Can you work these out from the model? Positions are in its coordinate system, mm. A direction names the side the tool comes from. Round coordinates to 2 decimals unless told otherwise and drop trailing zeros. Order: outer loops, then holes, each group sorted by start corner. A loop starts at its lowest first (then second) coordinate and runs counter-clockwise, first axis right, second up. Notation, with made-up numbers: M 53,84.5 L 80,84.5 A21 ccw 80,123.5 Z; hole C 58,66 d4. An arc over 180 degrees is marked long. Answer as a JSON object with one key per item and string values. Group by question number.
from build123d import *

# Parameters (mm, degrees)
SKETCH1_R          = 2.725
EXTRUDE1_DEPTH     = 2
CUT_EXTRUDE1_DEPTH = 1
SKETCH3_R          = 1.5
EXTRUDE2_DEPTH     = 20


with BuildPart() as part:
    # Sketch1 → Extrude1 (new body)
    with BuildSketch(Plane.XY):
        Circle(SKETCH1_R)
    extrude(amount=EXTRUDE1_DEPTH)

    # Sketch2 → Cut-Extrude1 (cut)
    with BuildSketch(Plane(origin=(0, 0, 0), x_dir=(-1, 0, 0), z_dir=(0, 0, -1))):
        Polygon((3.449801909, 0), (3.449801909, 0.55), (-3.901269584, 0.55), (-3.901269584, -0.55), (3.449801909, -0.55), align=None)
    extrude(amount=-CUT_EXTRUDE1_DEPTH, mode=Mode.SUBTRACT)

    # Sketch3 → Extrude2 (add)
    with BuildSketch(Plane.XY.offset(2)):
        Circle(SKETCH3_R)
    extrude(amount=EXTRUDE2_DEPTH)


solid = part.part
Item 1: On a 3-axis mill with a long thin cutter (end or side, diameter ignored), from which of +Z, -Z, +X, -X, +Y, -Y can I reach the whole of each face in a straight line? I mean faces 1 (the face through (0, -0.55, 0.5)), 2 (the face through (0, 0, 22)), 3 (the face through (-1.5, 0.07, 11.86)). Say none if no direction works.
Item 2: If we mould it in two halves opening along Y, with no side actions, what happens to faces 4 (the face through (0, 0, 1)), 5 (the face through (0, 0.55, 0.5)), 6 (the face through (1.2, -1.2, 2)), 7 (the face through (2.6, 0.82, 0.99))? For each: +Y half, -Y half, draft (parallel to the pull), parting line (faces both ways), or undercut.
Item 3: I'm going to push flat-ended pins straight in: pin 1 Ø2 at (x, y) = (0.5, 0) entering from -Z; pin 2 Ø2 at (x, z) = (0.5, 4.5) entering from -Y; pin 3 Ø1.5 at (y, z) = (-1.5, 15) entering from +X; pin 4 Ø1.5 at (y, z) = (2, 14) entering from -X. Where does each tip first touch, or does it pass through?
Item 4: Suppose I cut it at D-D, the plane y = -1.1. Write out the boundary of the cut face in (x, z).
Item 5: I need wall thicknesses on line 1 (Y direction, x = -0.1, z = 19.5); line 2 (Z direction, x = -1.25, y = 1); line 3 (Z direction, x = -0.65, y = -0.3). Which ranges of each line are inside material? Lowest first, please.
Item 6: Suppose I cut it at A-A, the plane x = 0. Write out the boundary of the cut face in (y, z) (3 decimals).
Item 7: Suppose I cut it at B-B, the plane y = 0. Write out the boundary of the cut face in (x, z) (3 decimals), and give its area (4 significant figures).
Item 8: Suppose I cut it at C-C, the plane z = 8.25. Write out the boundary of the cut face in (x, y), and give its area (3 significant figures).
Computed:
{
 "1": {"face 1": "-Z, +X, -X", "face 2": "+Z, +X, -X, +Y, -Y", "face 3": "+Z"},
 "2": {"face 4": "undercut", "face 5": "undercut", "face 6": "draft", "face 7": "parting line"},
 "3": {"pin 1": "stops at z = 0", "pin 2": "stops at y = -1.5", "pin 3": "stops at x = 1.3", "pin 4": "stops at x = -0.83"},
 "4": {"outline": "M -2.49,0 L 2.49,0 L 2.49,2 L 1.02,2 L 1.02,22 L -1.02,22 L -1.02,2 L -2.49,2 Z"},
 "5": {"line 1": "y = -1.5 to 1.5", "line 2": "z = 0 to 2", "line 3": "z = 1 to 22"},
 "6": {"outline": "M -2.725,0 L -0.55,0 L -0.55,1 L 0.55,1 L 0.55,0 L 2.725,0 L 2.725,2 L 1.5,2 L 1.5,22 L -1.5,22 L -1.5,2 L -2.725,2 Z"},
 "7": {"outline": "M -2.725,1 L 2.725,1 L 2.725,2 L 1.5,2 L 1.5,22 L -1.5,22 L -1.5,2 L -2.725,2 Z", "area": "65.45 mm^2"},
 "8": {"outline": "C 0,0 d3", "area": "7.07 mm^2"}
}
